Verification items for the finished model (mm, model axes). A direction names the side the tool comes from. Give positions to 0.01 mm unless a question says otherwise; leave off trailing zeros. Loops run counter-clockwise (first coordinate to the right, second up) from the corner with the lowest first, then second, coordinate; pieces in that order, holes last. Notation, with made-up numbers: M 84.5,86.5 L 105.5,86.5 A14 cw 105.5,101.5 Z; hole C -32.5,19.25 d7. An arc over 180 degrees is marked long. Answer in a Markdown table with one row per item.
```python
from build123d import *

# Parameters (mm, degrees)
SKETCH1_W               = 50
SKETCH1_H               = 15
BOSS_EXTRUDE1_DEPTH     = 5
CUT_EXTRUDE1_DEPTH      = 53.440442409
CUT_EXTRUDE1_DEPTH_BACK = 53.440442409
SKETCH2_R               = 1.5
SKETCH3_W               = 10
SKETCH3_H               = 5
CUT_EXTRUDE2_DEPTH      = 7.5
CUT_EXTRUDE3_DEPTH      = 53.440442409
CUT_EXTRUDE3_DEPTH_BACK = 53.440442409
SKETCH4_R               = 1.5


with BuildPart() as part:
    # Sketch1 → Boss-Extrude1 (new body)
    with BuildSketch(Plane(origin=(0, 0, 0), x_dir=(1, 0, 0), z_dir=(0, 1, 0))):
        with Locations((25, 7.5)):
            Rectangle(SKETCH1_W, SKETCH1_H)
    extrude(amount=BOSS_EXTRUDE1_DEPTH)

    # Sketch2 → Cut-Extrude1 (cut, two sides: drawn at the far end of the back side and taken through both)
    with BuildSketch(Plane(origin=(0, 5, 0), x_dir=(1, 0, 0), z_dir=(0, 1, 0)).offset(-CUT_EXTRUDE1_DEPTH_BACK)):
        with Locations(Location((5, 7.5, 0), (0, 0, 270))):
            Circle(SKETCH2_R)
    extrude(amount=CUT_EXTRUDE1_DEPTH + CUT_EXTRUDE1_DEPTH_BACK, mode=Mode.SUBTRACT)

    # Sketch3 → Cut-Extrude2 (cut)
    with BuildSketch(Plane(origin=(50, 0, 0), x_dir=(0, 0, -1), z_dir=(1, 0, 0))):
        with Locations((7.5, 2.5)):
            Rectangle(SKETCH3_W, SKETCH3_H)
    extrude(amount=-CUT_EXTRUDE2_DEPTH, mode=Mode.SUBTRACT)

    # Sketch4 → Cut-Extrude3 (cut, two sides: drawn at the far end of the back side and taken through both)
    with BuildSketch(Plane(origin=(0, 0, -15), x_dir=(-1, 0, 0), z_dir=(0, 0, -1)).offset(-CUT_EXTRUDE3_DEPTH_BACK)):
        with Locations(Location((-46.5, 2.5, 0), (0, 0, 90))):
            Circle(SKETCH4_R)
    extrude(amount=CUT_EXTRUDE3_DEPTH + CUT_EXTRUDE3_DEPTH_BACK, mode=Mode.SUBTRACT)


solid = part.part
```
Item 1: Sectioned sample at D-D (x = 5). Record the cut outline in (y, z), and give its area (3 significant figures).
Reported:
| item | result |
|---|---|
| outline | M 0,-15 L 5,-15 L 5,-9 L 0,-9 Z; M 0,-6 L 5,-6 L 5,0 L 0,0 Z |
| area | 60.0 mm^2 |
Item 2: Release check for a two-part mould opening along Z. For faces 3 (the cylindrical face through (5, 2, -9)), 4 (the flat face through (25, 2, 0)), 5 (the flat face through (25, 0, -8)) record: released by +Z, released by -Z, zero draft, split by the parting line, or undercut.
Reported:
| item | result |
|---|---|
| face 3 | undercut |
| face 4 | released by +Z |
| face 5 | zero draft |
Item 3: Sectioned sample at C-C (x = 46.5). Record the cut outline in (y, z).
Reported:
| item | result |
|---|---|
| outline | M 0,-15 L 1,-15 L 1,-12.5 L 0,-12.5 Z; M 0,-2.5 L 1,-2.5 L 1,0 L 0,0 Z; M 4,-15 L 5,-15 L 5,-12.5 L 4,-12.5 Z; M 4,-2.5 L 5,-2.5 L 5,0 L 4,0 Z |
Item 4: Go/stop test with flat-tipped pins: pin 1 (4 mm diameter, centred on x = 33, z = -8, fed in from -Y); pin 2 (3 mm diameter, centred on y = 2, z = -5.5, fed in from +X). Record where each tip stops, or that it passes through.
Reported:
| item | result |
|---|---|
| pin 1 | stops at y = 0 |
| pin 2 | stops at x = 42.5 |
Item 5: Scan lines: L1, parallel to X at y = 2.5, z = -0.95; L2, parallel to Z at x = 43.5, y = 1.9; L3, parallel to Z at x = 5, y = 3.05. Record each from-to range of solid material in increasing order. Write a range as [from, to].
Reported:
| item | result |
|---|---|
| L1 | x = [0, 45], [48, 50] |
| L2 | z = [-15, -12.5], [-2.5, 0] |
| L3 | z = [-15, -9], [-6, 0] |
Item 6: Sectioned sample at A-A (y = 2.5). Record the cut outline in (x, z).
Reported:
| item | result |
|---|---|
| outline | M 0,-15 L 45,-15 L 45,-12.5 L 42.5,-12.5 L 42.5,-2.5 L 45,-2.5 L 45,0 L 0,0 Z; M 48,-15 L 50,-15 L 50,-12.5 L 48,-12.5 Z; M 48,-2.5 L 50,-2.5 L 50,0 L 48,0 Z; hole C 5,-7.5 d3 |
Item 7: Sectioned sample at B-B (z = -7.5). Record the cut outline in (x, y).
Reported:
| item | result |
|---|---|
| outline | M 0,0 L 3.5,0 L 3.5,5 L 0,5 Z; M 6.5,0 L 42.5,0 L 42.5,5 L 6.5,5 Z |
Item 8: Tool access check on faces 1 (the flat face through (25, 5, -8)), 2 (the flat face through (45, 1, -2.5)). Record the directions out of +Z, -Z, +X, -X, +Y, -Y that give a thin tool (end or side, any length) a straight path to the whole face; none if there is none.
Reported:
| item | result |
|---|---|
| face 1 | +Z, -Z, +X, -X, +Y |
| face 2 | +X, +Y, -Y |
